Can you work these out from the drawing? Everything is in mm from the part's minimum corner. Coordinates: 2 decimals unless noted, no trailing zeros. Order: outer loops, then holes, each group sorted by start corner. A loop starts at its lowest first (then second) coordinate and runs counter-clockwise, first axis right, second up. Notation, with made-up numbers: (53.5, 61.25) - (110.5, 61.25) arc R17 cw to (110.5, 85.25) - close; hole circle Ø4 at (14, -25.75). An arc over 180 degrees is marked (long way). One line per item, written item: value.
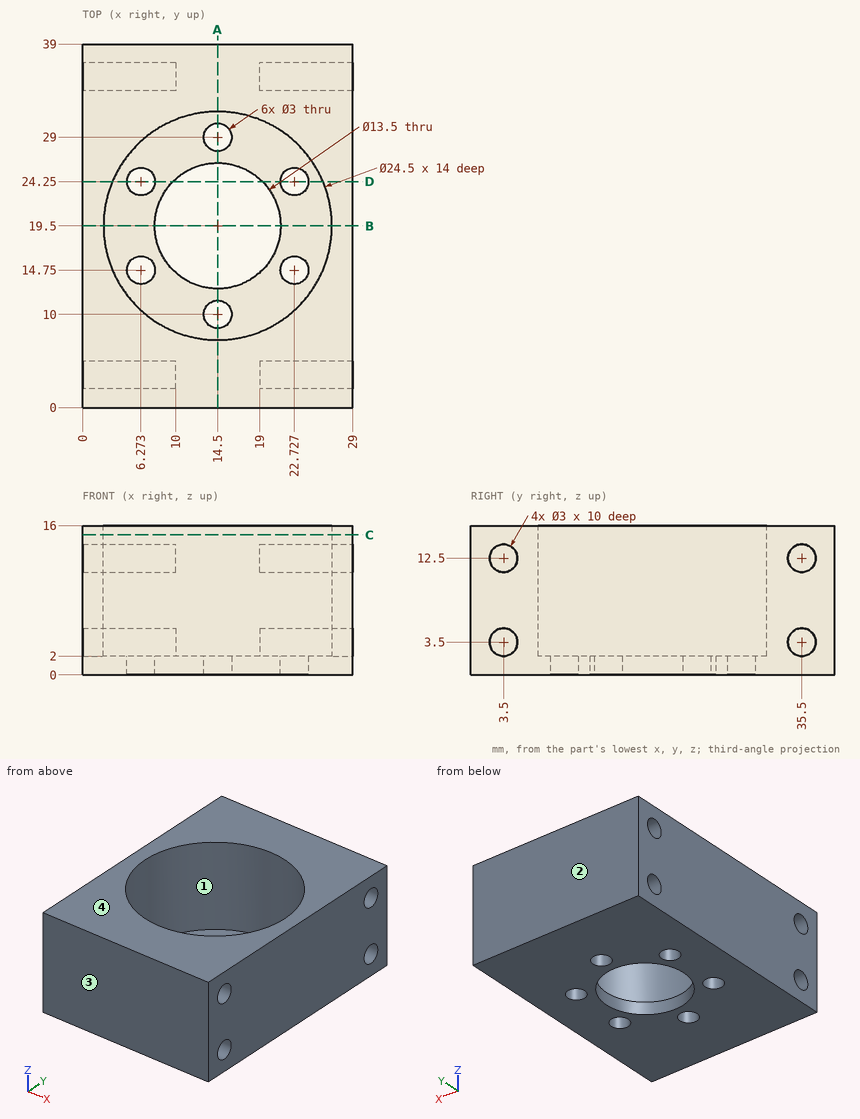
Item 1: I want a section at A-A on x = 14.5. Please give me the cut outline in (y, z).
Conclusion:
outline: (0, 0) - (8.5, 0) - (8.5, 2) - (7.25, 2) - (7.25, 16) - (0, 16) - close; (11.5, 0) - (12.75, 0) - (12.75, 2) - (11.5, 2) - close; (26.25, 0) - (27.5, 0) - (27.5, 2) - (26.25, 2) - close; (30.5, 0) - (39, 0) - (39, 16) - (31.75, 16) - (31.75, 2) - (30.5, 2) - close
Item 2: If I drill on probe 1 along Y at (x, z) = (27, 3.5); probe 2 along Y at (x, z) = (14.5, 1.25); probe 3 along Z at (x, y) = (5.5, 36) (1 decimal), over which ranges is the centre line in solid material (lowest first)?
Conclusion:
probe 1: 0 to 2, 5 to 34, 37 to 39
probe 2: 0 to 8.5, 11.5 to 12.75, 26.25 to 27.5, 30.5 to 39
probe 3: 0 to 2.1, 4.9 to 11.1, 13.9 to 16
Item 3: I want a section at C-C on z = 15. Please give me the cut outline in (x, y).
Conclusion:
outline: (0, 0) - (29, 0) - (29, 39) - (0, 39) - close; hole circle Ø24.5 at (14.5, 19.5)
Item 4: I want a section at D-D on y = 24.25. Please give me the cut outline in (x, z), then the cut area to 3 significant figures.
Conclusion:
outline: (0, 0) - (4.77, 0) - (4.77, 2) - (3.21, 2) - (3.21, 16) - (0, 16) - close; (7.77, 0) - (9.7, 0) - (9.7, 2) - (7.77, 2) - close; (19.3, 0) - (21.23, 0) - (21.23, 2) - (19.3, 2) - close; (24.23, 0) - (29, 0) - (29, 16) - (25.79, 16) - (25.79, 2) - (24.23, 2) - close
area: 117 mm²
Item 5: Thinking about a two-plate mould opening in Y: for the marked faces 1, 2, 3 and 4, which applies, pulls with the +Y half, pulls with the -Y half, needs draft (parallel to the pull), parting line crosses it, or undercut?
Conclusion:
face 1: undercut
face 2: pulls with the +Y half
face 3: pulls with the -Y half
face 4: needs draft
Item 6: I'm going to push flat-ended pins straight in: pin 1 Ø2.5 at (y, z) = (35.5, 3.5) entering from -X; pin 2 Ø0.9 at (y, z) = (35.5, 4) entering from +X; pin 3 Ø2.5 at (x, y) = (22.73, 14.75) entering from +Z. Where does each tip first touch, or does it pass through?
Conclusion:
pin 1: x = 10
pin 2: x = 19
pin 3: through
Item 7: I want a section at B-B on y = 19.5. Please give me the cut outline in (x, z).
Conclusion:
outline: (0, 0) - (7.75, 0) - (7.75, 2) - (2.25, 2) - (2.25, 16) - (0, 16) - close; (21.25, 0) - (29, 0) - (29, 16) - (26.75, 16) - (26.75, 2) - (21.25, 2) - close
